The listing builds one solid part. Answer for the finished solid, in the listing's coordinates (mm). Give positions to 0.01 mm unless a question says otherwise; leave off trailing zeros. Order: outer loops, then holes, each group sorted by start corner. A loop starts at its lowest first (then second) coordinate and runs counter-clockwise, first axis right, second up.
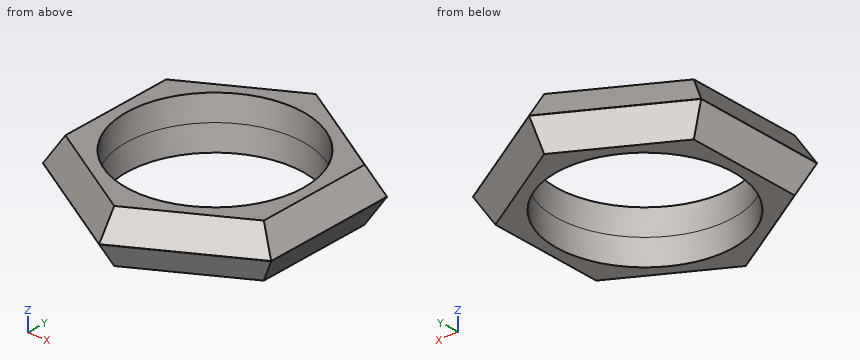
```python
from build123d import *

# Parameters (mm, degrees)
F0_R          = 8.6741
F1_DEPTH      = 2.54
F1_DEPTH_BACK = 2.54
F2_SIZE2      = 2.5296602045
F2_SIZE       = 1.4605
F3_SIZE2      = 2.5296602045
F3_SIZE       = 1.4605


with BuildPart() as f1:
    # F0 (on Top) → F1 (new body, two sides)
    with BuildSketch(Plane.XY) as f1_sk:
        Polygon((11.2141, -6.4744636537), (11.2141, 6.4744636537), (0, 12.9489273074), (-11.2141, 6.4744636537), (-11.2141, -6.4744636537), (0, -12.9489273074), align=None)
        Circle(F0_R, mode=Mode.SUBTRACT)
    extrude(amount=F1_DEPTH)
    extrude(f1_sk.sketch, amount=-F1_DEPTH_BACK)

    # F2
    f2_edges = [f1.edges().sort_by_distance(p)[0] for p in [
        (-5.60705, 9.711695, 2.54),
        (-11.2141, 0, 2.54),
        (-5.60705, -9.711695, 2.54),
        (5.60705, -9.711695, 2.54),
        (11.2141, 0, 2.54),
        (5.60705, 9.711695, 2.54),
    ]]
    f2_side = f1.faces().sort_by_distance((10.871504, 0, 2.54))[0]
    chamfer(f2_edges, length=F2_SIZE, length2=F2_SIZE2, reference=f2_side)

    # F3
    f3_edges = [f1.edges().sort_by_distance(p)[0] for p in [
        (-5.60705, 9.711695, -2.54),
        (-11.2141, 0, -2.54),
        (-5.60705, -9.711695, -2.54),
        (5.60705, -9.711695, -2.54),
        (11.2141, 0, -2.54),
        (5.60705, 9.711695, -2.54),
    ]]
    f3_side = f1.faces().sort_by_distance((10.871504, 0, -2.54))[0]
    chamfer(f3_edges, length=F3_SIZE, length2=F3_SIZE2, reference=f3_side)


solid = f1.part
```
1) Find section C-C (z = 2.1). Write down the section's boundary in (x, y).
Geometry says:
outline: (-10.01, -5.78) - (0, -11.56) - (10.01, -5.78) - (10.01, 5.78) - (0, 11.56) - (-10.01, 5.78) - close; hole circle Ø17.35 at (0, 0)
2) Given P1, Ø4, axis at x = 4, y = 5.5, coming from the +Z side; P2, Ø1.5, axis at y = -3.5, z = -2, coming from the -X side; P3, Ø10.5, axis at x = 0, y = 0, coming from the -Z side; P4, Ø2, axis at y = 3.5, z = 1.5, coming from the -X side, each flat-ended and moving along its own axis, determine where each tip first touches the part or whether it passes through.
Geometry says:
P1: stops at z = 2.54
P2: stops at x = -10.5
P3: passes through
P4: stops at x = -10.93
3) Straight lines are drawn through the part: probe 1 along Y at (x, z) = (-7.75, -1); probe 2 along X at (y, z) = (-6.75, 1.3); probe 3 along Y at (x, z) = (6.75, 1.75). For each, find the intervals that lie inside material, in ascending order.
Geometry says:
probe 1: y = -7.81 to -3.9, 3.9 to 7.81
probe 2: x = -9.25 to -5.45, 5.45 to 9.25
probe 3: y = -7.89 to -5.45, 5.45 to 7.89
